Can you work these out from the model? Positions are in its coordinate system, mm. A direction names the side the tool comes from. Round coordinates to 2 decimals unless told otherwise and drop trailing zeros. Loops run counter-clockwise (first coordinate to the right, second up) from the corner with the lowest first, then second, coordinate; pieces in that order, holes last. Notation, with made-up numbers: M -28.5,17.25 L 27.5,17.25 A18 ccw 27.5,30.25 Z; hole C -32.75,25.5 d9. An arc over 180 degrees is marked long. Return JSON: item names as keys, results as strings.
```python
from build123d import *

# Parameters (mm, degrees)
SKETCH_1_W          = 352
SKETCH_1_H          = 207
SKETCH_1_W_2        = 302
SKETCH_1_H_2        = 157
EXTRUDE_1_DEPTH     = 25
SKETCH_2_W          = 25
SKETCH_2_H          = 25
EXTRUDE_2_DEPTH     = 1045
SKETCH_3_W          = 352
SKETCH_3_H          = 207
SKETCH_3_W_2        = 302
SKETCH_3_H_2        = 157
EXTRUDE_3_DEPTH     = 25
EXTRUDE_START       = -25
SKETCH_4_W          = 302
SKETCH_4_H          = 25
EXTRUDE_4_DEPTH     = 25
SKETCH_5_W          = 302
SKETCH_5_H          = 25
EXTRUDE_5_DEPTH     = 25
SKETCH_6_W          = 25
SKETCH_6_H          = 25
EXTRUDE_6_DEPTH     = 150
CUT_EXTRUDE_1_REACH = 359
SKETCH_7_R          = 3


with BuildPart() as part:
    # Эскиз1 → Бобышка-Вытянуть1 (new body)
    with BuildSketch(Plane(origin=(0, 0, 0), x_dir=(1, 0, 0), z_dir=(0, 1, 0))):
        with Locations((176, 103.5)):
            Rectangle(SKETCH_1_W, SKETCH_1_H)
        with Locations((176, 103.5)):
            Rectangle(SKETCH_1_W_2, SKETCH_1_H_2, mode=Mode.SUBTRACT)
    extrude(amount=EXTRUDE_1_DEPTH)

    # Эскиз2 → Бобышка-Вытянуть2 (add)
    with BuildSketch(Plane(origin=(0, 25, 0), x_dir=(1, 0, 0), z_dir=(0, 1, 0))):
        with Locations((12.5, 194.5)):
            Rectangle(SKETCH_2_W, SKETCH_2_H)
        with Locations((12.5, 12.5)):
            Rectangle(SKETCH_2_W, SKETCH_2_H)
        with Locations((339.5, 12.5)):
            Rectangle(SKETCH_2_W, SKETCH_2_H)
        with Locations((339.5, 194.5)):
            Rectangle(SKETCH_2_W, SKETCH_2_H)
    extrude(amount=EXTRUDE_2_DEPTH)

    # Эскиз3 → Бобышка-Вытянуть3 (add)
    with BuildSketch(Plane(origin=(0, 1070, 0), x_dir=(1, 0, 0), z_dir=(0, 1, 0))):
        with Locations((176, 103.5)):
            Rectangle(SKETCH_3_W, SKETCH_3_H)
        with Locations((176, 103.5)):
            Rectangle(SKETCH_3_W_2, SKETCH_3_H_2, mode=Mode.SUBTRACT)
    extrude(amount=-EXTRUDE_3_DEPTH)

    # Эскиз4 → Бобышка-Вытянуть4 (add)
    with BuildSketch(Plane(origin=(0, 0, -207), x_dir=(-1, 0, 0), z_dir=(0, 0, -1)).offset(EXTRUDE_START)):
        with Locations((-176, 672.5)):
            Rectangle(SKETCH_4_W, SKETCH_4_H)
    extrude(amount=EXTRUDE_4_DEPTH)

    # Эскиз5 → Бобышка-Вытянуть5 (add)
    with BuildSketch(Plane.XY.offset(EXTRUDE_START)):
        with Locations((176, 537.5)):
            Rectangle(SKETCH_5_W, SKETCH_5_H)
    extrude(amount=EXTRUDE_5_DEPTH)

    # Эскиз6 → Бобышка-Вытянуть6 (add)
    with BuildSketch(Plane.XY):
        with Locations((339.5, 537.5)):
            Rectangle(SKETCH_6_W, SKETCH_6_H)
    extrude(amount=EXTRUDE_6_DEPTH)

    # Эскиз7 → Вырез-Вытянуть1 (cut, up to next)
    with BuildSketch(Plane(origin=(0, 0, -207), x_dir=(-1, 0, 0), z_dir=(0, 0, -1)), mode=Mode.PRIVATE) as cut_extrude_1_sk1:
        with Locations((-236, 672.5)):
            Circle(SKETCH_7_R)
    cut_extrude_1_tool1 = extrude(cut_extrude_1_sk1.sketch, amount=-CUT_EXTRUDE_1_REACH, mode=Mode.PRIVATE) & part.part
    add(cut_extrude_1_tool1.solids().sort_by_distance((236, 672.5, -207))[0], mode=Mode.SUBTRACT)
    # Эскиз7 → Вырез-Вытянуть1 (cut, up to next)
    with BuildSketch(Plane(origin=(0, 0, -207), x_dir=(-1, 0, 0), z_dir=(0, 0, -1)), mode=Mode.PRIVATE) as cut_extrude_1_sk2:
        with Locations((-116, 672.5)):
            Circle(SKETCH_7_R)
    cut_extrude_1_tool2 = extrude(cut_extrude_1_sk2.sketch, amount=-CUT_EXTRUDE_1_REACH, mode=Mode.PRIVATE) & part.part
    add(cut_extrude_1_tool2.solids().sort_by_distance((116, 672.5, -207))[0], mode=Mode.SUBTRACT)


solid = part.part
```
Q1. Suppose I cut it at B-B, the plane y = 344.5. Please give me the cut outline in (x, z).
Results:
{"outline": "M 0,-207 L 25,-207 L 25,-182 L 0,-182 Z; M 0,-25 L 25,-25 L 25,0 L 0,0 Z; M 327,-207 L 352,-207 L 352,-182 L 327,-182 Z; M 327,-25 L 352,-25 L 352,0 L 327,0 Z"}
Q2. If I drill on line 1 along Y through (x, z) = (236, -187.75); line 2 along X through (y, z) = (672.5, -190.25), over which ranges is the centre line in solid material (lowest first)?
Results:
{"line 1": "y = 0 to 25, 660 to 669.5, 675.5 to 685, 1045 to 1070", "line 2": "x = 0 to 113, 119 to 233, 239 to 352"}
Q3. I'm going to push flat-ended pins straight in: pin 1 Ø7.5 at (y, z) = (16, -86) entering from -X; pin 2 Ø12.5 at (x, y) = (139, 1061.5) entering from +Z; pin 3 Ø20 at (y, z) = (542.5, 51) entering from -X. Where does each tip first touch, or does it pass through?
Results:
{"pin 1": "stops at x = 0", "pin 2": "stops at z = 0", "pin 3": "stops at x = 327"}
Q4. Thinking about a two-plate mould opening in Y: for faces 6 (the flat face through (174, 550, -13)), 7 (the flat face through (174, 1070, -197)), 8 (the flat face through (339, 538, 150)), which applies, pulls with the +Y half, pulls with the -Y half, needs draft (parallel to the pull), parting line crosses it, or undercut?
Results:
{"face 6": "undercut", "face 7": "pulls with the +Y half", "face 8": "needs draft"}
Q5. Suppose I cut it at A-A, the plane x = 201. Please give me the cut outline in (y, z).
Results:
{"outline": "M 0,-207 L 25,-207 L 25,-182 L 0,-182 Z; M 0,-25 L 25,-25 L 25,0 L 0,0 Z; M 525,-25 L 550,-25 L 550,0 L 525,0 Z; M 660,-207 L 685,-207 L 685,-182 L 660,-182 Z; M 1045,-207 L 1070,-207 L 1070,-182 L 1045,-182 Z; M 1045,-25 L 1070,-25 L 1070,0 L 1045,0 Z"}
Q6. Suppose I cut it at C-C, the plane z = -96. Please give me the cut outline in (x, y), plus the area to 3 significant figures.
Results:
{"outline": "M 0,0 L 25,0 L 25,25 L 0,25 Z; M 0,1045 L 25,1045 L 25,1070 L 0,1070 Z; M 327,0 L 352,0 L 352,25 L 327,25 Z; M 327,1045 L 352,1045 L 352,1070 L 327,1070 Z", "area": "2,500 mm2"}
Q7. On a 3-axis mill with a long thin cutter (end or side, diameter ignored), from which of +Z, -Z, +X, -X, +Y, -Y can I reach the whole of each face in a straight line? I mean faces 1 (the flat face through (174, 12, -25)), 2 (the flat face through (352, 533, -16)), 3 (the flat face through (175, 684, -182)), 4 (the flat face through (327, 537, 74)), 5 (the flat face through (174, 1045, -13)). Say none if no direction works.
Results:
{"face 1": "+Y, -Y", "face 2": "+Z, -Z, +X, +Y, -Y", "face 3": "+X, -X", "face 4": "+Z, -X, +Y, -Y", "face 5": "+Z, -Z"}
